from build123d import *

# Parameters (mm, degrees)
F3_W     = 1.6
F3_H     = 96.388348
F4_R     = 5.2
F5_R     = 4.05
F8_DEPTH = 5.201


with BuildPart() as f6:
    # F6: sweep along a path in F1
    with BuildLine(Plane.XZ) as f6_path:
        Line((0, 0), (0, 0.6))
        Line((0, 0.6), (0, 3.2))
    # F2 (on Top) + F3 (on Top) → F6 (sweep)
    with BuildSketch(Plane.XY):
        with BuildLine():
            ThreePointArc((49.794174, 44.194174), (48.153972, 48.153972), (44.194174, 49.794174))
            Line((44.194174, 49.794174), (0, 49.794174))
            Line((0, 49.794174), (-44.194174, 49.794174))
            ThreePointArc((-44.194174, 49.794174), (-48.153972, 48.153972), (-49.794174, 44.194174))
            Line((-49.794174, 44.194174), (-49.794174, 0))
            Line((-49.794174, 0), (-49.794174, -44.194174))
            ThreePointArc((-49.794174, -44.194174), (-48.153972, -48.153972), (-44.194174, -49.794174))
            Line((-44.194174, -49.794174), (0, -49.794174))
            Line((0, -49.794174), (44.194174, -49.794174))
            ThreePointArc((44.194174, -49.794174), (48.153972, -48.153972), (49.794174, -44.194174))
            Line((49.794174, -44.194174), (49.794174, 0))
            Line((49.794174, 0), (49.794174, 44.194174))
        make_face()
        with BuildLine():
            Line((0, 48.194174), (40.27499, 48.194174))
            ThreePointArc((40.27499, 48.194174), (40.234376, 40.234376), (48.194174, 40.27499))
            Line((48.194174, 40.27499), (48.194174, 0))
            Line((48.194174, 0), (48.194174, -40.27499))
            ThreePointArc((48.194174, -40.27499), (40.234376, -40.234376), (40.27499, -48.194174))
            Line((40.27499, -48.194174), (0, -48.194174))
            Line((0, -48.194174), (-40.27499, -48.194174))
            ThreePointArc((-40.27499, -48.194174), (-40.234376, -40.234376), (-48.194174, -40.27499))
            Line((-48.194174, -40.27499), (-48.194174, 0))
            Line((-48.194174, 0), (-48.194174, 40.27499))
            ThreePointArc((-48.194174, 40.27499), (-40.234376, 40.234376), (-40.27499, 48.194174))
            Line((-40.27499, 48.194174), (0, 48.194174))
        make_face(mode=Mode.SUBTRACT)
    with BuildSketch(Plane.XY):
        with Locations((-13.3, 0)):
            Rectangle(F3_W, F3_H)
        with Locations((13.3, 0)):
            Rectangle(F3_W, F3_H)
    sweep(path=f6_path.line)

    # F7: sweep along a path in F1
    with BuildLine(Plane.XZ) as f7_path:
        Line((0, 0), (0, 0.6))
        Line((0, 0.6), (0, 3.2))
        Line((0, 3.2), (0, 5.2))
    # F4 (on Top) → F7 (sweep)
    with BuildSketch(Plane.XY):
        with Locations((44.194174, 44.194174)):
            Circle(F4_R)
        with Locations((-44.194174, 44.194174)):
            Circle(F4_R)
        with Locations((-44.194174, -44.194174)):
            Circle(F4_R)
        with Locations((44.194174, -44.194174)):
            Circle(F4_R)
    sweep(path=f7_path.line)

    # F5 (on Top) → F8 (cut, through all)
    with BuildSketch(Plane.XY):
        with Locations((44.194174, 44.194174)):
            Circle(F5_R)
        with Locations((-44.194174, 44.194174)):
            Circle(F5_R)
        with Locations((-44.194174, -44.194174)):
            Circle(F5_R)
        with Locations((44.194174, -44.194174)):
            Circle(F5_R)
    extrude(amount=F8_DEPTH, mode=Mode.SUBTRACT)


solid = f6.part
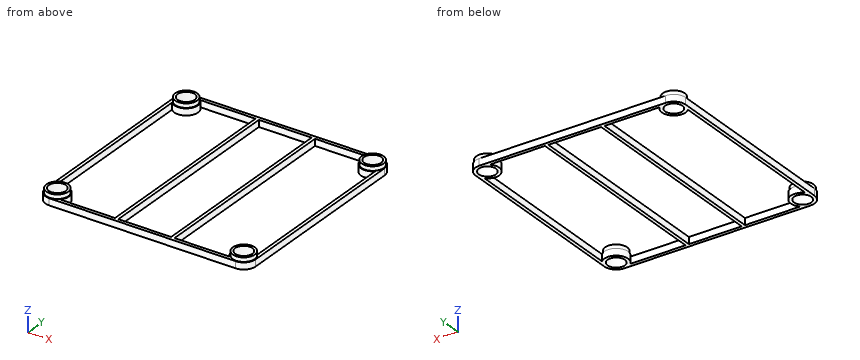
Check sheet for the modelled part. Datum: model origin and axes. Units: mm. Coordinates: 2 decimals unless noted, no trailing zeros. Loops run counter-clockwise (first coordinate to the right, second up) from the corner with the lowest first, then second, coordinate; pieces in that order, holes last. Notation, with made-up numbers: (16.5, -33) -> (38.5, -33) arc R14 ccw to (38.5, -13) -> close; hole circle Ø8 at (28.25, 62.25). An arc over 180 degrees is marked (long way). Answer in a Markdown table with one row per item.
1. Sectioned sample at A-A, the plane z = 4.4. Record the boundary of the cut face in (x, y).
Check values:
| item | result |
|---|---|
| outline | circle Ø10.4 at (-44.19, -44.19); circle Ø10.4 at (-44.19, 44.19); circle Ø10.4 at (44.19, -44.19); circle Ø10.4 at (44.19, 44.19); hole circle Ø8.1 at (-44.19, -44.19); hole circle Ø8.1 at (-44.19, 44.19); hole circle Ø8.1 at (44.19, -44.19); hole circle Ø8.1 at (44.19, 44.19) |
2. Sectioned sample at C-C, the plane y = -15. Record the boundary of the cut face in (x, z), then the cut area to 3 significant figures.
Check values:
| item | result |
|---|---|
| outline | (-49.79, 0) -> (-48.19, 0) -> (-48.19, 3.2) -> (-49.79, 3.2) -> close; (-14.1, 0) -> (-12.5, 0) -> (-12.5, 3.2) -> (-14.1, 3.2) -> close; (12.5, 0) -> (14.1, 0) -> (14.1, 3.2) -> (12.5, 3.2) -> close; (48.19, 0) -> (49.79, 0) -> (49.79, 3.2) -> (48.19, 3.2) -> close |
| area | 20.5 mm2 |
3. Sectioned sample at B-B, the plane x = 5.5. Record the boundary of the cut face in (y, z), then the cut area to 3 significant figures.
Check values:
| item | result |
|---|---|
| outline | (-49.79, 0) -> (-48.19, 0) -> (-48.19, 3.2) -> (-49.79, 3.2) -> close; (48.19, 0) -> (49.79, 0) -> (49.79, 3.2) -> (48.19, 3.2) -> close |
| area | 10.2 mm2 |
4. Go/stop test with flat-tipped pins: pin 1 (5 mm diameter, centred on x = 44.19, y = -44.19, fed in from -Z); pin 2 (10 mm diameter, centred on x = -18.5, y = 29.5, fed in from +Z). Record where each tip stops, or that it passes through.
Check values:
| item | result |
|---|---|
| pin 1 | passes through |
| pin 2 | stops at z = 3.2 |
5. Material ranges on line 1 along X through (y, z) = (27, 3.05); line 2 along Y through (x, z) = (15.5, 2.85); line 3 along Y through (x, z) = (41.5, 4.35), recorded low to high. Write a range as [from, to].
Check values:
| item | result |
|---|---|
| line 1 | x = [-49.79, -48.19], [-14.1, -12.5], [12.5, 14.1], [48.19, 49.79] |
| line 2 | y = [-49.79, -48.19], [48.19, 49.79] |
| line 3 | y = [-48.64, -47.22], [-41.17, -39.75], [39.75, 41.17], [47.22, 48.64] |
